```python
from build123d import *

# Parameters (mm, degrees)
BOSS_EXTRUDE1_DEPTH = 12.7
SKETCH2_R           = 1.500000048
CUT_EXTRUDE1_DEPTH  = 58.854101994
FILLET1_R           = 7.62
CUT_EXTRUDE2_DEPTH  = 62.533611452
BOSS_EXTRUDE2_DEPTH = 2.54


with BuildPart() as part:
    # Sketch1 → Boss-Extrude1 (new body)
    with BuildSketch(Plane(origin=(0, 0, 0), x_dir=(1, 0, 0), z_dir=(0, 1, 0))):
        with BuildLine():
            ThreePointArc((12.7, -54.091601994), (0, -55.5625), (-12.7, -54.091601994))
            Line((-12.7, -54.091601994), (-12.7, -58.854101994))
            Line((-12.7, -58.854101994), (12.7, -58.854101994))
            Line((12.7, -58.854101994), (12.7, -54.091601994))
        make_face()
    extrude(amount=BOSS_EXTRUDE1_DEPTH)

    # Sketch2 → Cut-Extrude1 (cut)
    with BuildSketch(Plane.XY):
        with Locations(Location((-7.62, 7.62, 0), (0, 0, 180))):
            Circle(SKETCH2_R)
    cut_extrude1 = extrude(amount=CUT_EXTRUDE1_DEPTH, mode=Mode.SUBTRACT)

    # Mirror1: Cut-Extrude1 across plane
    add(cut_extrude1.mirror(Plane(origin=(0, 0, 0), x_dir=(0, 0, 1), z_dir=(1, 0, 0))), mode=Mode.SUBTRACT)

    # Fillet1
    fillet1_edges = [part.edges().sort_by_distance(p)[0] for p in [
        (-12.7, 0, 56.472851994),
        (12.7, 0, 56.472851994),
    ]]
    fillet(fillet1_edges, radius=FILLET1_R)

    # Sketch2<4> → Cut-Extrude2 (cut, through all)
    with BuildSketch(Plane.XY):
        with BuildLine():
            ThreePointArc((1.549999948, 3.81), (1.096015474, 4.906015474), (0, 5.359999948))
            Line((0, 5.359999948), (0, 2.260000052))
            ThreePointArc((0, 2.260000052), (1.096015474, 2.713984526), (1.549999948, 3.81))
        make_face()
        with BuildLine():
            Line((0, 2.260000052), (0, 5.359999948))
            ThreePointArc((0, 5.359999948), (-1.549999948, 3.81), (0, 2.260000052))
        make_face()
    extrude(amount=CUT_EXTRUDE2_DEPTH, mode=Mode.SUBTRACT)

    # Sketch7 → Boss-Extrude2 (add)
    with BuildSketch(Plane(origin=(0, 12.7, 0), x_dir=(1, 0, 0), z_dir=(0, 1, 0))):
        with BuildLine():
            Line((-12.7, -54.091601994), (-12.7, -58.854101994))
            Line((-12.7, -58.854101994), (12.7, -58.854101994))
            Line((12.7, -58.854101994), (12.7, -54.091601994))
            ThreePointArc((12.7, -54.091601994), (0, -55.5625), (-12.7, -54.091601994))
        make_face()
        with BuildLine():
            ThreePointArc((-12.7, -47.545558744), (0, -49.2125), (12.7, -47.545558744))
            Line((12.7, -47.545558744), (12.7, -54.091601994))
            ThreePointArc((12.7, -54.091601994), (0, -55.5625), (-12.7, -54.091601994))
            Line((-12.7, -54.091601994), (-12.7, -47.545558744))
        make_face()
    extrude(amount=BOSS_EXTRUDE2_DEPTH)


solid = part.part
```
Build history of the part. All positions in model axes, mm. A direction names the side the tool comes from. Coordinates: 2 decimals unless noted, no trailing zeros. Order: outer loops, then holes, each group sorted by start corner. A loop starts at its lowest first (then second) coordinate and runs counter-clockwise, first axis right, second up.
Item 1: Saw through at A-A on z = 57. List the corners of the cut face in (x, y), then the cut area to 3 significant figures.
Filled in:
outline: (-12.7, 7.62) arc R7.62 ccw to (-5.08, 0) - (5.08, 0) arc R7.62 ccw to (12.7, 7.62) - (12.7, 15.24) - (-12.7, 15.24) - close; hole circle Ø3 at (-7.62, 7.62); hole circle Ø3.1 at (0, 3.81); hole circle Ø3 at (7.62, 7.62)
area: 340 mm2
Item 2: Drop flat-ended pins along their axis: pin 1 Ø1.5 at (x, y) = (4.5, 9) entering from -Z; pin 2 Ø1.5 at (y, z) = (5.5, 57.5) entering from +X; pin 3 Ø2.5 at (x, z) = (6, 50.5) entering from -Y. Give the stop position or say it passes through.
Filled in:
pin 1: stops at z = 55.31
pin 2: stops at x = 12.58
pin 3: stops at y = 12.7
Item 3: Saw through at B-B on x = -8.75. List the corners of the cut face in (y, z).
Filled in:
outline: (0.94, 54.87) - (6.63, 54.87) - (6.63, 58.85) - (0.94, 58.85) - close; (8.61, 54.87) - (12.7, 54.87) - (12.7, 48.43) - (15.24, 48.43) - (15.24, 58.85) - (8.61, 58.85) - close
Item 4: Tool access for faces 1 (the flat face through (0, 12.7, 51)), 2 (the flat face through (0, 8, 58.854)): list every direction of +Z, -Z, +X, -X, +Y, -Y with a clear straight run to the whole face (end or side of a thin tool).
Filled in:
face 1: -Z, -Y
face 2: +Z, +X, -X, +Y, -Y
Item 5: Drill centre lines: L1, parallel to X at y = 7.62, z = 56.9; L2, parallel to Z at x = -1.5, y = 9.5; L3, parallel to Y at x = 7.62, z = 56.5. Where is each one in solid material? Low to high.
Filled in:
L1: x = -12.7 to -9.12, -6.12 to 6.12, 9.12 to 12.7
L2: z = 55.54 to 58.85
L3: y = 0.44 to 6.12, 9.12 to 15.24
Item 6: Saw through at D-D on x = -3.25. List the corners of the cut face in (y, z), then the cut area to 3 significant figures.
Filled in:
outline: (0, 55.47) - (12.7, 55.47) - (12.7, 49.11) - (15.24, 49.11) - (15.24, 58.85) - (0, 58.85) - close
area: 67.8 mm2
Item 7: Saw through at C-C on y = 3.5. List the corners of the cut face in (x, z) (1 decimal), then the cut area to 3 significant figures.
Filled in:
outline: (-11.5, 54.4) arc R55.6 cw to (-1.5, 55.5) - (-1.5, 58.9) - (-11.5, 58.9) - close; (1.5, 55.5) arc R55.6 cw to (11.5, 54.4) - (11.5, 58.9) - (1.5, 58.9) - close
area: 74.8 mm2
Item 8: Mould opens along X. For faces 3 (the flat face through (-12.7, 12.2, 54.4)), 4 (the cylindrical face through (-0.18, 13.952, 49.212)), 5 (the flat face through (0, 15.24, 53)) say: released by +X, released by -X, zero draft, split by the parting line, or undercut.
Filled in:
face 3: released by -X
face 4: undercut
face 5: zero draft
